Can you work these out from the model? Positions are in its coordinate system, mm. Face numbers are marked on the shaded views. A direction names the side the tool comes from. Round coordinates to 2 decimals unless told otherwise and drop trailing zeros. Order: outer loops, then holes, each group sorted by start corner. A loop starts at its lowest first (then second) coordinate and runs counter-clockwise, first axis right, second up. Notation, with made-up numbers: M 69,38.5 L 128,38.5 A28 ccw 128,76.5 Z; hole C -22.75,-21 d10. An arc over 180 degrees is marked long. Answer as a JSON object with one key per item and string values. Group by question number.
```python
from build123d import *

# Parameters (mm, degrees)
M16X2_0_TAPPED_HOLE1_D = 14
SKETCH4_W              = 21
SKETCH4_H              = 8
CUT_EXTRUDE1_DEPTH     = 8
CHAMFER2_SIZE          = 2


with BuildPart() as part:
    # Sketch1 → Revolve1 (revolve)
    with BuildSketch(Plane.XY, mode=Mode.PRIVATE) as revolve1_sk:
        Polygon((-40, 25), (40, 25), (45, 25), (45, 37.5), (40, 37.5), (40, 108), (15, 108), (15, 50), (-40, 50), align=None)
    revolve(revolve1_sk.sketch.rotate(Axis((-40, 0, 0), (1, 0, 0)), 90), axis=Axis((-40, 0, 0), (1, 0, 0)))

    # M16x2.0 Tapped Hole1 (through all)
    with Locations(Plane(origin=(40, 0, 0), x_dir=(0, 0, -1), z_dir=(1, 0, 0))):
        with Locations((-75, 0), (0, 75), (75, 0), (0, -75)):
            Hole(M16X2_0_TAPPED_HOLE1_D / 2)

    # Sketch4 → Revolve2 (revolve)
    with BuildSketch(Plane.XY, mode=Mode.PRIVATE) as revolve2_sk:
        with Locations((4.5, 104)):
            Rectangle(SKETCH4_W, SKETCH4_H)
    revolve(revolve2_sk.sketch.rotate(Axis((0, 0, 0), (1, 0, 0)), 90), axis=Axis((0, 0, 0), (1, 0, 0)))

    # Sketch5 → Cut-Extrude1 (cut, symmetric)
    with BuildSketch(Plane.XY):
        Polygon((-40, 0), (45, 0), (45, 28.4), (-40, 27.55), align=None)
    extrude(amount=CUT_EXTRUDE1_DEPTH, both=True, mode=Mode.SUBTRACT)

    # Chamfer2
    chamfer2_edges = [part.edges().sort_by_distance(p)[0] for p in [
        (45, 0, -37.5),
        (-6, 0, -108),
        (-40, 0, -50),
        (15, 0, -50),
    ]]
    chamfer(chamfer2_edges, length=CHAMFER2_SIZE)


solid = part.part
```
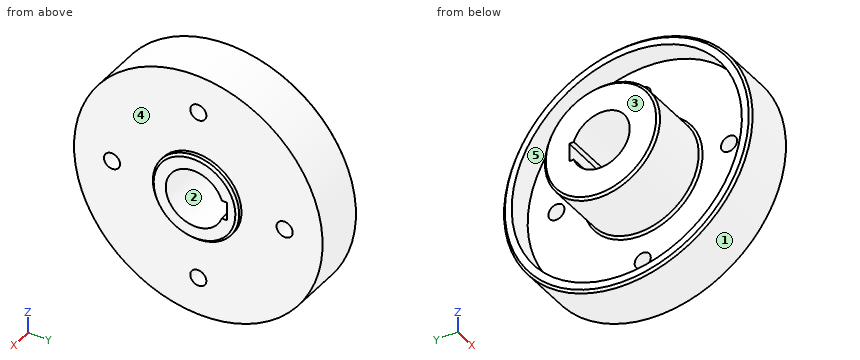
1) For pin 1 (5 mm diameter, centred on x = 25.5, z = -59, fed in from +Y); pin 2 (1 mm diameter, centred on y = 80, z = 17.5, fed in from -X); pin 3 (4 mm diameter, centred on y = 13.5, z = 54, fed in from +X); pin 4 (11 mm diameter, centred on y = -75, z = 0, fed in from -X), each with a flat end and sliding along its axis, tell me the tip position at first contact or that it passes through.
2) We'd pull the mould along Y, two halves only. Please class the marked faces 1, 2 and 3: +Y half, -Y half, draft (parallel to the pull), parting line (faces both ways), or undercut.
3) I need wall thicknesses on line 1 along Y through (x, z) = (-5, -3); line 2 along Z through (x, y) = (8, -32.5); line 3 along Y through (x, z) = (29.5, 0) (3 decimals). Which ranges of each line are inside material? Lowest first, please.
4) If we section it at B-B on z = 0: Count the separate pieces of the cut face and the enclosed holes in it, plus the area to 3 significant figures.
5) If we section it at A-A on x = 18: Write out the boundary of the cut face in (y, z), plus the area to 3 significant figures.
6) If we section it at D-D on x = -26.5: Write out the boundary of the cut face in (y, z) (3 decimals).
7) Which directions (+Z, -Z, +X, -X, +Y, -Y) give clear straight access to the entire face, cutting with the end or side of a thin tool? Please do the marked faces 4 and 5.
Findings:
{
 "1": {"pin 1": "stops at y = 92.04", "pin 2": "stops at x = 15", "pin 3": "stops at x = 40", "pin 4": "passes through"},
 "2": {"face 1": "parting line", "face 2": "undercut", "face 3": "draft"},
 "3": {"line 1": "y = -106.96 to -99.95, -49.91 to -24.82, 27.9 to 49.91, 99.95 to 106.96", "line 2": "z = -102.99 to -94.57, -38 to 38, 94.57 to 102.99", "line 3": "y = -108 to -82, -68 to -25, 28.245 to 68, 82 to 108"},
 "4": {"separate pieces": "4", "enclosed holes": "0", "area": "6,400 mm^2"},
 "5": {"outline": "C 0,0 d216; hole C -75,0 d14; hole C 0,-75 d14; hole C 0,75 d14; hole M 23.69,-8 L 28.13,-8 L 28.13,8 L 23.69,8 A25 ccw long Z; hole C 75,0 d14", "area": "34,000 mm^2"},
 "6": {"outline": "C 0,0 d100; hole M 23.685,-8 L 27.685,-8 L 27.685,8 L 23.685,8 A25 ccw long Z"},
 "7": {"face 4": "+X", "face 5": "-X"}
}
